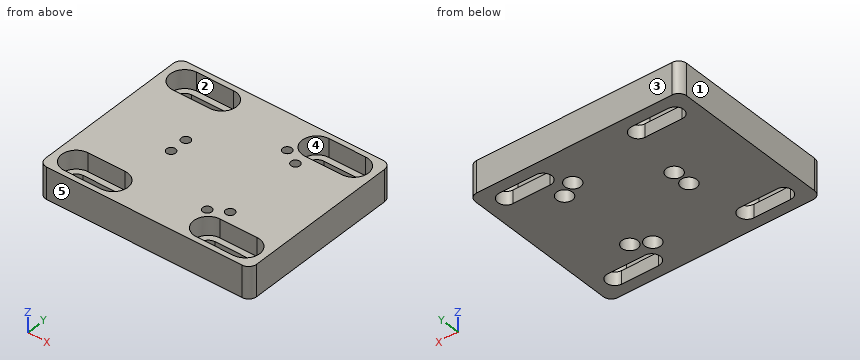
```python
from build123d import *

# Parameters (mm, degrees)
SKETCH_1_W          = 80
SKETCH_1_H          = 65
SKETCH_1_R          = 1.7
SKETCH_1_R_2        = 3.2
EXTRUDE_1_DEPTH     = 12
SKETCH_2_R          = 3
CUT_EXTRUDE_1_DEPTH = 9.4
FILLET_1_R          = 3
CUT_EXTRUDE_2_DEPTH = 7
CUT_EXTRUDE_3_DEPTH = 53.012017842


with BuildPart() as part:
    # 스케치1 → 보스-돌출1 (new body)
    with BuildSketch(Plane.XY):
        Rectangle(SKETCH_1_W, SKETCH_1_H)
        with Locations((-13.82389773, -3.407324542)):
            Circle(SKETCH_1_R, mode=Mode.SUBTRACT)
        with Locations((-13.82389773, 3.407324542)):
            Circle(SKETCH_1_R, mode=Mode.SUBTRACT)
        with Locations((18.112778477, 15.031324063)):
            Circle(SKETCH_1_R, mode=Mode.SUBTRACT)
        with Locations((12.211119252, 18.438648605)):
            Circle(SKETCH_1_R, mode=Mode.SUBTRACT)
        with Locations((12.211119252, -18.438648605)):
            Circle(SKETCH_1_R, mode=Mode.SUBTRACT)
        with Locations((18.112778477, -15.031324063)):
            Circle(SKETCH_1_R, mode=Mode.SUBTRACT)
        with Locations((25, -25)):
            Circle(SKETCH_1_R_2, mode=Mode.SUBTRACT)
        with Locations((25, 25)):
            Circle(SKETCH_1_R_2, mode=Mode.SUBTRACT)
        with Locations((-25, 25)):
            Circle(SKETCH_1_R_2, mode=Mode.SUBTRACT)
        with Locations((-25, -25)):
            Circle(SKETCH_1_R_2, mode=Mode.SUBTRACT)
    extrude(amount=EXTRUDE_1_DEPTH)

    # 스케치2 → 컷-돌출1 (cut)
    with BuildSketch(Plane(origin=(0, 0, 0), x_dir=(-1, 0, 0), z_dir=(0, 0, -1))):
        with Locations((-12.211119252, 18.438648605)):
            Circle(SKETCH_2_R)
        with Locations((-18.112778477, 15.031324063)):
            Circle(SKETCH_2_R)
        with Locations((-12.211119252, -18.438648605)):
            Circle(SKETCH_2_R)
        with Locations((-18.112778477, -15.031324063)):
            Circle(SKETCH_2_R)
        with Locations((13.82389773, -3.407324542)):
            Circle(SKETCH_2_R)
        with Locations((13.82389773, 3.407324542)):
            Circle(SKETCH_2_R)
    extrude(amount=-CUT_EXTRUDE_1_DEPTH, mode=Mode.SUBTRACT)

    # 필렛1
    fillet_1_edges = [part.edges().sort_by_distance(p)[0] for p in [
        (40, 32.5, 6),
        (40, -32.5, 6),
        (-40, -32.5, 6),
        (-40, 32.5, 6),
    ]]
    fillet(fillet_1_edges, radius=FILLET_1_R)

    # 스케치3 → 컷-돌출2 (cut)
    with BuildSketch(Plane.XY.offset(12)):
        with BuildLine():
            Line((-32, 30.5), (-18, 30.5))
            ThreePointArc((-18, 30.5), (-12.5, 25), (-18, 19.5))
            Line((-18, 19.5), (-32, 19.5))
            ThreePointArc((-32, 19.5), (-37.5, 25), (-32, 30.5))
        make_face()
        with BuildLine():
            Line((32, 19.5), (18, 19.5))
            ThreePointArc((18, 19.5), (12.5, 25), (18, 30.5))
            Line((18, 30.5), (32, 30.5))
            ThreePointArc((32, 30.5), (37.5, 25), (32, 19.5))
        make_face()
        with BuildLine():
            Line((32, -30.5), (18, -30.5))
            ThreePointArc((18, -30.5), (12.5, -25), (18, -19.5))
            Line((18, -19.5), (32, -19.5))
            ThreePointArc((32, -19.5), (37.5, -25), (32, -30.5))
        make_face()
        with BuildLine():
            Line((-32, -19.5), (-18, -19.5))
            ThreePointArc((-18, -19.5), (-12.5, -25), (-18, -30.5))
            Line((-18, -30.5), (-32, -30.5))
            ThreePointArc((-32, -30.5), (-37.5, -25), (-32, -19.5))
        make_face()
    extrude(amount=-CUT_EXTRUDE_2_DEPTH, mode=Mode.SUBTRACT)

    # 스케치4 → 컷-돌출3 (cut, through all)
    with BuildSketch(Plane.XY.offset(5)):
        with BuildLine():
            Line((-32, 28.2), (-18, 28.2))
            ThreePointArc((-18, 28.2), (-14.8, 25), (-18, 21.8))
            Line((-18, 21.8), (-32, 21.8))
            ThreePointArc((-32, 21.8), (-35.2, 25), (-32, 28.2))
        make_face()
        with BuildLine():
            Line((18, 28.2), (32, 28.2))
            ThreePointArc((32, 28.2), (35.2, 25), (32, 21.8))
            Line((32, 21.8), (18, 21.8))
            ThreePointArc((18, 21.8), (14.8, 25), (18, 28.2))
        make_face()
        with BuildLine():
            Line((32, -28.2), (18, -28.2))
            ThreePointArc((18, -28.2), (14.8, -25), (18, -21.8))
            Line((18, -21.8), (32, -21.8))
            ThreePointArc((32, -21.8), (35.2, -25), (32, -28.2))
        make_face()
        with BuildLine():
            Line((-32, -21.8), (-18, -21.8))
            ThreePointArc((-18, -21.8), (-14.8, -25), (-18, -28.2))
            Line((-18, -28.2), (-32, -28.2))
            ThreePointArc((-32, -28.2), (-35.2, -25), (-32, -21.8))
        make_face()
    extrude(amount=-CUT_EXTRUDE_3_DEPTH, mode=Mode.SUBTRACT)


solid = part.part
```
Can you work these out from the model? Positions are in its coordinate system, mm. Face numbers are marked on the shaded views. A direction names the side the tool comes from. Round coordinates to 2 decimals unless told otherwise and drop trailing zeros. Order: outer loops, then holes, each group sorted by start corner. A loop starts at its lowest first (then second) coordinate and runs counter-clockwise, first axis right, second up. Notation, with made-up numbers: (19, -33.75) -> (59, -33.75) arc R11 ccw to (59, -22.75) -> close; hole circle Ø9 at (86, -39.5). An arc over 180 degrees is marked (long way). Return JSON: item names as keys, results as strings. Group by question number.
1. If we section it at A-A, the plane y = 25: Write out the boundary of the cut face in (x, z).
2. If we section it at C-C, the plane y = -24: Write out the boundary of the cut face in (x, z).
3. We'd pull the mould along Y, two halves only. Please class the marked faces 1, 2 and 3: released by +Y, released by -Y, zero draft, split by the parting line, or undercut.
4. If we section it at B-B, the plane z = 11: Count the separate pieces of the cut face and the enclosed holes in it, then the cut area to 3 significant figures.
5. Will these pins go through, and if not, where does the flat tip stop? pin 1 (5.5 mm diameter, centred on x = 26.5, y = 27.5, fed in from +Z); pin 2 (1.8 mm diameter, centred on x = 11, y = -17.5, fed in from -Z); pin 3 (2 mm diameter, centred on x = 12.21, y = -18.44, fed in from +Z); pin 4 (7 mm diameter, centred on x = -13.82, y = 3.41, fed in from +Z).
6. Which directions (+Z, -Z, +X, -X, +Y, -Y) give clear straight access to the entire face, cutting with the end or side of a thin tool? Please do the marked faces 4 and 5.
7. I need wall thicknesses on line 1 (Y direction, x = -21, z = 5.5); line 2 (Y direction, x = -26, z = 4.5); line 3 (Y direction, x = 13.5, z = 7). Which ranges of each line are inside material? Lowest first, please. Write a range as [from, to].
Output values:
{
 "1": {"outline": "(-40, 0) -> (-35.2, 0) -> (-35.2, 5) -> (-37.5, 5) -> (-37.5, 12) -> (-40, 12) -> close; (-14.8, 0) -> (14.8, 0) -> (14.8, 5) -> (12.5, 5) -> (12.5, 12) -> (-12.5, 12) -> (-12.5, 5) -> (-14.8, 5) -> close; (35.2, 0) -> (40, 0) -> (40, 12) -> (37.5, 12) -> (37.5, 5) -> (35.2, 5) -> close"},
 "2": {"outline": "(-40, 0) -> (-35.04, 0) -> (-35.04, 5) -> (-37.41, 5) -> (-37.41, 12) -> (-40, 12) -> close; (-14.96, 0) -> (14.96, 0) -> (14.96, 5) -> (12.59, 5) -> (12.59, 12) -> (-12.59, 12) -> (-12.59, 5) -> (-14.96, 5) -> close; (35.04, 0) -> (40, 0) -> (40, 12) -> (37.41, 12) -> (37.41, 5) -> (35.04, 5) -> close"},
 "3": {"face 1": "zero draft", "face 2": "undercut", "face 3": "released by +Y"},
 "4": {"separate pieces": "1", "enclosed holes": "10", "area": "4,140 mm²"},
 "5": {"pin 1": "z = 5", "pin 2": "z = 9.4", "pin 3": "through", "pin 4": "z = 12"},
 "6": {"face 4": "+Z", "face 5": "+Z, -Z, +X, -X, -Y"},
 "7": {"line 1": "[-32.5, -30.5], [-19.5, 19.5], [30.5, 32.5]", "line 2": "[-32.5, -28.2], [-21.8, 21.8], [28.2, 32.5]", "line 3": "[-32.5, -28.16], [-21.84, -21.15], [-15.73, 15.73], [21.15, 21.84], [28.16, 32.5]"}
}
